Input: part model. Units: mm. Frame: model coordinates. Face numbers are marked on the shaded views. A direction names the side the tool comes from. Coordinates: 2 decimals unless noted, no trailing zeros. Order: outer loops, then holes, each group sorted by start corner. A loop starts at its lowest first (then second) coordinate and runs counter-clockwise, first axis right, second up.
from build123d import *

# Parameters (mm, degrees)
F4_W      = 91
F4_H      = 218
F5_DEPTH  = 41
F8_DEPTH  = 218
F9_DEPTH  = 91
F10_W     = 85
F10_H     = 212
F11_DEPTH = 38
F12_R     = 0.75


with BuildPart() as f5:
    # F4 (on Top) → F5 (new body)
    with BuildSketch(Plane.XY):
        with Locations((45.5, 109)):
            Rectangle(F4_W, F4_H)
    extrude(amount=F5_DEPTH)

    # F7 (on face) → F8 (join)
    with BuildSketch(Plane.XZ):
        Polygon((0, 44), (0, 41), (1.5, 41), (3, 44), align=None)
    extrude(amount=-F8_DEPTH)

    # F6 (on face) → F9 (join)
    with BuildSketch(Plane.YZ.offset(91)):
        Polygon((0, 44), (0, 41), (1.5, 41), (3, 44), align=None)
        Polygon((216.5, 41), (218, 41), (218, 44), (215, 44), align=None)
    extrude(amount=-F9_DEPTH)

    # F10 (on face) → F11 (cut)
    with BuildSketch(Plane.XY.offset(41)):
        with Locations((45.5, 109)):
            Rectangle(F10_W, F10_H)
    extrude(amount=-F11_DEPTH, mode=Mode.SUBTRACT)

    # F12
    f12_edges = [f5.edges().sort_by_distance(p)[0] for p in [
        (91, 0, 22),
        (91, 218, 22),
        (0, 0, 22),
    ]]
    fillet(f12_edges, radius=F12_R)

    # F13 (on face) → F14 (revolve)
    with BuildSketch(Plane.XY.offset(41)):
        with BuildLine():
            Line((88.5, 109), (90.5, 109))
            ThreePointArc((90.5, 109), (89.5, 110), (88.5, 109))
        make_face()
    revolve(axis=Axis((24.0288835471, 109, 41), (-1, 0, 0)))


solid = f5.part
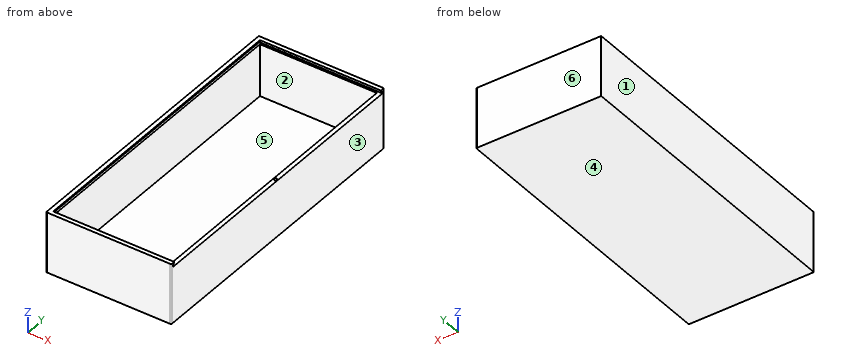
Item 1: Cut plane C-C on x = 6. Return loops of the section in (y, z).
Response values:
outline: (0, 0) - (218, 0) - (218, 44) - (215, 44) - (216.5, 41) - (215, 41) - (215, 3) - (3, 3) - (3, 41) - (1.5, 41) - (3, 44) - (0, 44) - close
Item 2: Cut plane B-B on z = 15.5. Return loops of the section in (x, y), then the cut area to 3 significant figures.
Response values:
outline: (0, 0.75) arc R0.75 ccw to (0.75, 0) - (90.25, 0) arc R0.75 ccw to (91, 0.75) - (91, 217.25) arc R0.75 ccw to (90.25, 218) - (0, 218) - close; hole (3, 3) - (88, 3) - (88, 215) - (3, 215) - close
area: 1,820 mm2
Item 3: Draft query along X for the marked faces 1, 2, 3 and 4. Return one class per face: pulls with the +X half, pulls with the -X half, needs draft (parallel to the pull), parting line crosses it, or undercut.
Response values:
face 1: pulls with the -X half
face 2: undercut
face 3: pulls with the +X half
face 4: needs draft
Item 4: Access query for the marked faces 5 and 6. Directions: +Z, -Z, +X, -X, +Y, -Y. A direction counts if a zero-diameter tool reaches every point of the face in a straight line with its end or side. Return the directions, or none.
Response values:
face 5: +Z
face 6: +Z, -Z, +X, -X, +Y
Item 5: Cut plane A-A on y = 183.5. Return loops of the section in (x, z).
Response values:
outline: (0, 0) - (91, 0) - (91, 41) - (88, 41) - (88, 3) - (3, 3) - (3, 41) - (1.5, 41) - (3, 44) - (0, 44) - close
Item 6: Ray query, probe 1 along X at (y, z) = (26, 23); probe 2 along Y at (x, z) = (55, 38); probe 3 along Z at (x, y) = (10, 162). Return the intervals inside material, ascending.
Response values:
probe 1: x = 0 to 3, 88 to 91
probe 2: y = 0 to 3, 215 to 218
probe 3: z = 0 to 3
